Read the model definition and answer for the solid it produces. Units are mm, in the model's axes. Give positions to 0.01 mm unless a question says otherwise; leave off trailing zeros. Loops run counter-clockwise (first coordinate to the right, second up) from the corner with the lowest first, then second, coordinate; pieces in that order, holes last. Notation, with made-up numbers: (77, 32.25) - (135, 32.25) arc R25 cw to (135, 68.25) - close; hole circle Ø9 at (-10, 71). An arc over 180 degrees is marked (long way). Use a Markdown table: item, result. Add a question column.
Item 1: Each of these flat-tipped pins is pushed along its axis until it touches: P1, Ø1.5, axis at x = 0.5, z = 8.5, coming from the +Y side; P2, Ø3, axis at x = 0, y = 0, coming from the +Z side; P3, Ø3, axis at x = -2, z = 22, coming from the -Y side. Where does it stop, or does it pass through?
Item 2: Consider probe 1 along X at (y, z) = (0, 23.75); probe 2 along X at (y, z) = (-0.75, 26.5); probe 3 along Y at (x, z) = (0, -22.5). Determine where each line is inside the solid, lowest interval first. Write a range as [from, to].
Item 3: A cutting plane is placed at A-A (z = -20.5). Determine the outline of the cut face in (x, y).
Item 4: A cutting plane is placed at B-B (z = 0.5). Determine the outline of the cut face in (x, y), plus the area to 3 significant figures.
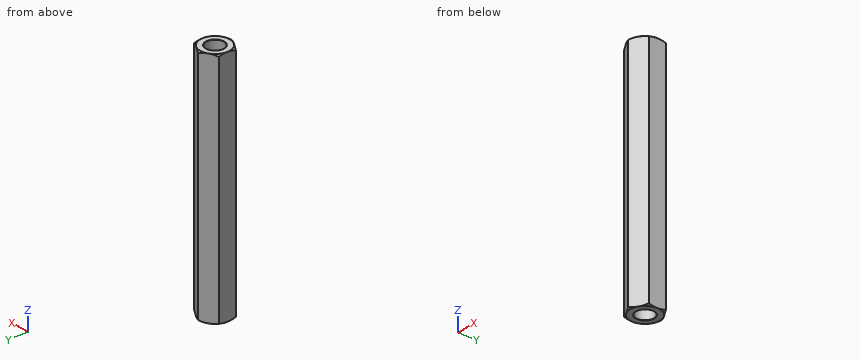
from build123d import *

# Parameters (mm, degrees)
EXTRUDE1_DEPTH          = 31.75
EXTRUDE1_DEPTH_BACK     = 31.75
SKETCH1_R               = 2.413
SKETCH8_OUTSIDE_W       = 247.302
SKETCH8_OUTSIDE_H       = 248.53
SKETCH8_OUTSIDE_R       = 3.96875
EXTRUDE4_DEPTH          = 64.788731596
EXTRUDE4_DRAFT          = -60
MIRROR1_COPY_1_SKETCH_W = 247.302
MIRROR1_COPY_1_SKETCH_H = 248.53
MIRROR1_COPY_1_SKETCH_R = 3.96875
MIRROR1_COPY_1_DEPTH    = 64.788731596
MIRROR1_COPY_1_DRAFT    = -60
SKETCH9_W               = 38.1
SKETCH9_H               = 2.4638


with BuildPart() as part:
    # Sketch1 → Extrude1 (new, two sides: drawn at the far end of the back side and taken through both)
    with BuildSketch(Plane.XY.offset(-EXTRUDE1_DEPTH_BACK)):
        Polygon((0, 4.582717762), (-3.96875, 2.291358881), (-3.96875, -2.291358881), (0, -4.582717762), (3.96875, -2.291358881), (3.96875, 2.291358881), align=None)
        Circle(SKETCH1_R, mode=Mode.SUBTRACT)
    extrude(amount=EXTRUDE1_DEPTH + EXTRUDE1_DEPTH_BACK)

    # Extrude3 cone 1 section (through the dimple's axis) → Extrude3 (revolve, cut)
    with BuildSketch(Plane(origin=(0, 0, -31.75), x_dir=(0, 1, 0), z_dir=(1, 0, 0))):
        Polygon((0, 0), (2.4638, 0), (0, 2.642102028), align=None)
    extrude3 = revolve(axis=Axis((0, 0, -31.75), (0, 0, 1)), mode=Mode.SUBTRACT)


with BuildPart() as extrude4_tool:
    # Sketch8 outside → Extrude4 (with draft: the straight prism first)
    with BuildSketch(Plane(origin=(0, 0, -31.75), x_dir=(-1, 0, 0), z_dir=(0, 0, -1))):
        Rectangle(SKETCH8_OUTSIDE_W, SKETCH8_OUTSIDE_H)
        Circle(SKETCH8_OUTSIDE_R, mode=Mode.SUBTRACT)
    extrude(amount=-EXTRUDE4_DEPTH)
    # Extrude4: the draft: its side faces are tilted about the plane it starts from
    extrude4_sides = [extrude4_tool.faces().sort_by_distance(p)[0] for p in [
        (0, -124.265, 0.644365798),
        (-123.651, 0, 0.644365798),
        (0, 124.265, 0.644365798),
        (123.651, 0, 0.644365798),
        (3.96875, 0, 0.644365798),
    ]]
    draft(extrude4_sides, Plane(origin=(0, 0, -31.75), x_dir=(-1, 0, 0), z_dir=(0, 0, -1)), EXTRUDE4_DRAFT)


with BuildPart() as part_1:
    add(part.part)

    # Extrude4: cut by extrude4_tool
    add(extrude4_tool.part, mode=Mode.SUBTRACT)

    # Mirror1: Extrude3 across plane
    add(extrude3.mirror(Plane.XY), mode=Mode.SUBTRACT)


with BuildPart() as mirror1_copy_1_tool:
    # Mirror1 copy 1 sketch → Mirror1 copy 1 (with draft: the straight prism first)
    with BuildSketch(Plane(origin=(0, 0, 31.75), x_dir=(-1, 0, 0), z_dir=(0, 0, 1))):
        Rectangle(MIRROR1_COPY_1_SKETCH_W, MIRROR1_COPY_1_SKETCH_H)
        Circle(MIRROR1_COPY_1_SKETCH_R, mode=Mode.SUBTRACT)
    extrude(amount=-MIRROR1_COPY_1_DEPTH)
    # Mirror1 copy 1: the draft: its side faces are tilted about the plane it starts from
    mirror1_copy_1_sides = [mirror1_copy_1_tool.faces().sort_by_distance(p)[0] for p in [
        (0, -124.265, -0.644365798),
        (-123.651, 0, -0.644365798),
        (0, 124.265, -0.644365798),
        (123.651, 0, -0.644365798),
        (3.96875, 0, -0.644365798),
    ]]
    draft(mirror1_copy_1_sides, Plane(origin=(0, 0, 31.75), x_dir=(-1, 0, 0), z_dir=(0, 0, 1)), MIRROR1_COPY_1_DRAFT)


with BuildPart() as part_2:
    add(part_1.part)

    # Mirror1 copy 1: cut by mirror1_copy_1_tool
    add(mirror1_copy_1_tool.part, mode=Mode.SUBTRACT)

    # Sketch9 → Revolve 2 (revolve)
    with BuildSketch(Plane(origin=(0, 0, 0), x_dir=(0, 0, -1), z_dir=(1, 0, 0)), mode=Mode.PRIVATE) as revolve_2_sk:
        with Locations((0, 1.2319)):
            Rectangle(SKETCH9_W, SKETCH9_H)
    revolve(revolve_2_sk.sketch.rotate(Axis((0, 0, 31.75), (0, 0, -1)), 270), axis=Axis((0, 0, 31.75), (0, 0, -1)))


solid = part_2.part
Geometry says:
| question | item | result |
|---|---|---|
| 1 | P1 | y = 4.58 |
| 1 | P2 | z = 19.05 |
| 1 | P3 | y = -4.29 |
| 2 | probe 1 | [-3.97, -2.41], [2.41, 3.97] |
| 2 | probe 2 | [-3.97, -2.29], [2.29, 3.97] |
| 2 | probe 3 | [-4.58, -2.41], [2.41, 4.58] |
| 3 | outline | (-3.97, -2.29) - (0, -4.58) - (3.97, -2.29) - (3.97, 2.29) - (0, 4.58) - (-3.97, 2.29) - close; hole circle Ø4.83 at (0, 0) |
| 4 | outline | (-3.97, -2.29) - (0, -4.58) - (3.97, -2.29) - (3.97, 2.29) - (0, 4.58) - (-3.97, 2.29) - close |
| 4 | area | 54.6 mm² |
